```python
from build123d import *

# Parameters (mm, degrees)
F0_W     = 139.7
F0_H     = 25.4
F1_DEPTH = 50.8
F2_R     = 5.08
F3_R     = 0.79375
F4_DEPTH = 20.32
F5_W     = 3.175
F5_H     = 12.7
F6_DEPTH = 12.7
F7_R     = 1.5875
F8_DEPTH = 20.32


with BuildPart() as f1:
    # F0 (on Front) → F1 (new body)
    with BuildSketch(Plane.XZ):
        with Locations((-0.889001, -1.383466)):
            Rectangle(F0_W, F0_H)
    extrude(amount=F1_DEPTH)

    # F2
    f2_edges = [f1.edges().sort_by_distance(p)[0] for p in [
        (-70.739001, -25.4, 11.316534),
        (-70.739001, -25.4, -14.083466),
        (68.960999, -25.4, 11.316534),
        (68.960999, -25.4, -14.083466),
    ]]
    fillet(f2_edges, radius=F2_R)

    # F3 (on face) → F4 (cut)
    with BuildSketch(Plane.XY.offset(11.316534)):
        with Locations((-51.373154, -7.14375)):
            Circle(F3_R)
        with Locations((-51.373154, -43.65625)):
            Circle(F3_R)
    extrude(amount=-F4_DEPTH, mode=Mode.SUBTRACT)

    # F5 (on face) → F6 (cut)
    with BuildSketch(Plane.XY.offset(11.316534)):
        with Locations((-15.614189, -25.083785)):
            Rectangle(F5_W, F5_H)
    extrude(amount=-F6_DEPTH, mode=Mode.SUBTRACT)

    # F7 (on face) → F8 (cut)
    with BuildSketch(Plane.XY.offset(11.316534)):
        with Locations((0, -11.1125)):
            Circle(F7_R)
        with Locations((0, -39.6875)):
            Circle(F7_R)
    extrude(amount=-F8_DEPTH, mode=Mode.SUBTRACT)


solid = f1.part
```
The listing builds one solid part. Answer for the finished solid, in the listing's coordinates (mm). A direction names the side the tool comes from. Give positions to 0.01 mm unless a question says otherwise; leave off trailing zeros. Order: outer loops, then holes, each group sorted by start corner. A loop starts at its lowest first (then second) coordinate and runs counter-clockwise, first axis right, second up. Notation, with made-up numbers: (73, -27) -> (104, -27) arc R25 ccw to (104, -3) -> close; hole circle Ø3 at (-6.5, 38). An arc over 180 degrees is marked (long way). Answer as a JSON object with one key per item and string values. Group by question number.
Item 1: Consider L1, parallel to Y at x = 0, z = -4 (3 decimals); L2, parallel to X at y = -30, z = 1.5; L3, parallel to X at y = -21, z = 9. Determine where each line is inside the solid, lowest interval first. Write a range as from..to.
Item 2: The part is cut by section C-C on z = -12.25. Write down the section's boundary in (x, y), and give its area (3 significant figures).
Item 3: A flat-ended cylindrical pin translates along its axis: pin 1 (1 mm diameter, centred on x = 0.5, y = -11.5, fed in from +Z). Find the tip coordinate at first contact, or state that the pin passes through.
Item 4: A tool of negligible diameter and unlimited length cuts with its end or side. For faces 1 (the flat face through (-16, -31.434, 5)), 2 (the flat face through (-2, 0, -1)), from which of +Z, -Z, +X, -X, +Y, -Y can it reach the whole face along a straight path? Write none if from no direction.
Item 5: The part is cut by section A-A on y = -27.5. Write down the section's boundary in (x, z), and give its area (3 significant figures).
Item 6: Determine the mould class of faces 3 (the cylindrical face through (67.433, -25.756, -12.635)), 4 (the flat face through (-16, -25, -1.383)), 5 (the flat face through (-2, -25, -14.083)) for opening direction X: pulls with the +X half, pulls with the -X half, needs draft (parallel to the pull), parting line crosses it, or undercut.
Item 7: The part is cut by section B-B on x = 0. Write down the section's boundary in (y, z) (3 decimals).
Result set:
{
 "1": {"L1": "-50.8..-41.275, -38.1..-12.7, -9.525..0", "L2": "-70.74..-17.2, -14.03..68.96", "L3": "-69.92..-17.2, -14.03..68.14"},
 "2": {"outline": "(-69.57, -50.8) -> (67.79, -50.8) -> (67.79, 0) -> (-69.57, 0) -> close", "area": "6,980 mm²"},
 "3": {"pin 1": "z = -9"},
 "4": {"face 1": "+Z", "face 2": "+Z, -Z, +X, -X, +Y"},
 "5": {"outline": "(-70.74, -9) arc R5.08 ccw to (-65.66, -14.08) -> (63.88, -14.08) arc R5.08 ccw to (68.96, -9) -> (68.96, 6.24) arc R5.08 ccw to (63.88, 11.32) -> (-14.03, 11.32) -> (-14.03, -1.38) -> (-17.2, -1.38) -> (-17.2, 11.32) -> (-65.66, 11.32) arc R5.08 ccw to (-70.74, 6.24) -> close", "area": "3,490 mm²"},
 "6": {"face 3": "pulls with the +X half", "face 4": "undercut", "face 5": "needs draft"},
 "7": {"outline": "(-50.8, -14.083) -> (0, -14.083) -> (0, 11.317) -> (-9.525, 11.317) -> (-9.525, -9.003) -> (-12.7, -9.003) -> (-12.7, 11.317) -> (-38.1, 11.317) -> (-38.1, -9.003) -> (-41.275, -9.003) -> (-41.275, 11.317) -> (-50.8, 11.317) -> close"}
}
